Could you check a few things on this model? Use its own coordinates, in mm. A direction names the side the tool comes from. Coordinates: 2 decimals unless noted, no trailing zeros. Write each loop counter-clockwise with the first axis right and the second up, starting at its lowest first coordinate (ties: lowest second). Pieces come first, ordered by that corner, then holes. Notation, with made-up numbers: (65, 24) - (124, 24) arc R31 ccw to (124, 48) - close; hole circle Ø8 at (-1.75, 81). An arc over 180 degrees is marked (long way). Answer as a JSON object with one key per item and string values. Group by question number.
1) Will these pins go through, and if not, where does the flat tip stop? pin 1 Ø4 at (y, z) = (-12, 6) entering from -X; pin 2 Ø8 at (x, y) = (7.5, -2) entering from -Z; pin 3 Ø8 at (y, z) = (-20.5, 14.5) entering from -X; pin 4 Ø2.5 at (y, z) = (0, 17.5) entering from -X.
2) On a 3-axis mill with a long thin cutter (end or side, diameter ignored), from which of +Z, -Z, +X, -X, +Y, -Y can I reach the whole of each face in a straight line? I mean faces 4 (the cylindrical face through (-9.151, -0.088, 15.502)), 5 (the flat face through (12.1, -22.3, 1.5)), 6 (the cylindrical face through (-1.2, -9.2, 15.9)), 7 (the cylindrical face through (3.252, 14.643, 17.404)). Say none if no direction works.
3) If we section it at D-D (y = -7.5): Write out the boundary of the cut face in (x, z).
4) If we section it at A-A (y = 0): Write out the boundary of the cut face in (x, z), plus the area to 3 significant figures.
5) We'd pull the mould along Z, two halves only. Please class faces 1 (the flat face through (12, -12, 14.2)), 2 (the flat face through (0, -6, 0)), 3 (the cylindrical face through (-20, -15.33, 7.02)): released by +Z, released by -Z, zero draft, split by the parting line, or undercut.
6) If we section it at C-C (z = 17.5): Write out the boundary of the cut face in (x, y), plus the area to 3 significant figures.
7) Please list where these lines run through material, in increasing order: line 1 along Z through (x, y) = (0, -6); line 2 along Z through (x, y) = (-17, -21); line 3 along X through (y, z) = (3, 9).
```python
from build123d import *

# Parameters (mm, degrees)
CROQUIS1_R              = 27.55
SALIENTE_EXTRUIR1_DEPTH = 1.5
CROQUIS2_R              = 25.2
SALIENTE_EXTRUIR2_DEPTH = 11.2
CROQUIS3_R              = 27.55
SALIENTE_EXTRUIR3_DEPTH = 1.5
CROQUIS8_R              = 15
SALIENTE_EXTRUIR5_DEPTH = 6.5
CROQUIS6_R              = 2
CORTAR_EXTRUIR3_DEPTH   = 45.119100172
CROQUIS5_R              = 2
CORTAR_EXTRUIR2_DEPTH   = 45.119100219
CROQUIS4_R              = 4
CORTAR_EXTRUIR1_DEPTH   = 45.119100172


with BuildPart() as part:
    # Croquis1 → Saliente-Extruir1 (new body)
    with BuildSketch(Plane.XY):
        Circle(CROQUIS1_R)
    extrude(amount=SALIENTE_EXTRUIR1_DEPTH)

    # Croquis2 → Saliente-Extruir2 (add)
    with BuildSketch(Plane.XY.offset(1.5)):
        Circle(CROQUIS2_R)
    extrude(amount=SALIENTE_EXTRUIR2_DEPTH)

    # Croquis3 → Saliente-Extruir3 (add)
    with BuildSketch(Plane.XY.offset(12.7)):
        Circle(CROQUIS3_R)
    extrude(amount=SALIENTE_EXTRUIR3_DEPTH)

    # Croquis8 → Saliente-Extruir5 (add)
    with BuildSketch(Plane.XY.offset(14.2)):
        with Locations(Location((0, 0, 0), (0, 0, 180))):
            Circle(CROQUIS8_R)
    extrude(amount=SALIENTE_EXTRUIR5_DEPTH)

    # Croquis6 → Cortar-Extruir3 (cut, through all)
    with BuildSketch(Plane(origin=(0, 0, 0), x_dir=(1, 0, 0), z_dir=(0, 1, 0))):
        with Locations(Location((0, -17.5, 0), (0, 0, 270))):
            Circle(CROQUIS6_R)
    extrude(amount=-CORTAR_EXTRUIR3_DEPTH, mode=Mode.SUBTRACT)

    # Croquis5 → Cortar-Extruir2 (cut, through all)
    with BuildSketch(Plane(origin=(0, 0, 0), x_dir=(0, 0, -1), z_dir=(1, 0, 0))):
        with Locations(Location((-17.5, 0, 0), (0, 0, 180))):
            Circle(CROQUIS5_R)
    extrude(amount=-CORTAR_EXTRUIR2_DEPTH, mode=Mode.SUBTRACT)

    # Croquis4 → Cortar-Extruir1 (cut, through all)
    with BuildSketch(Plane.XY.offset(20.7)):
        Circle(CROQUIS4_R)
    extrude(amount=-CORTAR_EXTRUIR1_DEPTH, mode=Mode.SUBTRACT)


solid = part.part
```
Here are the results:
{
 "1": {"pin 1": "stops at x = -23.13", "pin 2": "stops at z = 0", "pin 3": "stops at x = -22.05", "pin 4": "stops at x = 3.8"},
 "2": {"face 4": "-X", "face 5": "none", "face 6": "-Y", "face 7": "+Z"},
 "3": {"outline": "(-26.51, 0) - (26.51, 0) - (26.51, 1.5) - (24.06, 1.5) - (24.06, 12.7) - (26.51, 12.7) - (26.51, 14.2) - (12.99, 14.2) - (12.99, 20.7) - (-12.99, 20.7) - (-12.99, 14.2) - (-26.51, 14.2) - (-26.51, 12.7) - (-24.06, 12.7) - (-24.06, 1.5) - (-26.51, 1.5) - close; hole circle Ø4 at (0, 17.5)"},
 "4": {"outline": "(-27.55, 0) - (-4, 0) - (-4, 15.5) - (-15, 15.5) - (-15, 14.2) - (-27.55, 14.2) - (-27.55, 12.7) - (-25.2, 12.7) - (-25.2, 1.5) - (-27.55, 1.5) - close; (-15, 19.5) - (-4, 19.5) - (-4, 20.7) - (-15, 20.7) - close; (4, 0) - (27.55, 0) - (27.55, 1.5) - (25.2, 1.5) - (25.2, 12.7) - (27.55, 12.7) - (27.55, 14.2) - (15, 14.2) - (15, 20.7) - (4, 20.7) - close", "area": "715 mm²"},
 "5": {"face 1": "released by +Z", "face 2": "released by -Z", "face 3": "undercut"},
 "6": {"outline": "(-14.87, -2) arc R15 ccw to (-2, -14.87) - (-2, -3.46) arc R4 cw to (-3.46, -2) - close; (-14.87, 2) - (-3.46, 2) arc R4 cw (long way) to (2, -3.46) - (2, -14.87) arc R15 ccw (long way) to start", "area": "568 mm²"},
 "7": {"line 1": "z = 0 to 15.5, 19.5 to 20.7", "line 2": "z = 0 to 1.5, 12.7 to 14.2", "line 3": "x = -25.02 to -2.65, 2.65 to 25.02"}
}
